```python
from build123d import *

# Parameters (mm, degrees)
BOX002_W     = 24
BOX002_H     = 2.4
BOX002_DEPTH = 20
BOX003_W     = 24
BOX003_H     = 2.4
BOX003_DEPTH = 20
BOX004_W     = 24
BOX004_H     = 2.4
BOX004_DEPTH = 20
BOX001_W     = 24
BOX001_H     = 2.4
BOX001_DEPTH = 20
BOX_W        = 30
BOX_H        = 33
BOX_DEPTH    = 22


with BuildPart() as box002:
    # Box002 → Box002 (new body)
    with BuildSketch(Plane(origin=(0, 5.6, 0), x_dir=(1, 0, 0), z_dir=(0, 0, 1))):
        with Locations((12, 1.2)):
            Rectangle(BOX002_W, BOX002_H)
    extrude(amount=BOX002_DEPTH)


with BuildPart() as box003:
    # Box003 → Box003 (new body)
    with BuildSketch(Plane(origin=(0, 11.2, 0), x_dir=(1, 0, 0), z_dir=(0, 0, 1))):
        with Locations((12, 1.2)):
            Rectangle(BOX003_W, BOX003_H)
    extrude(amount=BOX003_DEPTH)


with BuildPart() as box004:
    # Box004 → Box004 (new body)
    with BuildSketch(Plane(origin=(0, 16.8, 0), x_dir=(1, 0, 0), z_dir=(0, 0, 1))):
        with Locations((12, 1.2)):
            Rectangle(BOX004_W, BOX004_H)
    extrude(amount=BOX004_DEPTH)


with BuildPart() as ranuras:
    # Box001 → Box001 (new body)
    with BuildSketch(Plane.XY):
        with Locations((12, 1.2)):
            Rectangle(BOX001_W, BOX001_H)
    extrude(amount=BOX001_DEPTH)

    # Fusion: union Box002, Box003, Box004
    add(box002.part)
    add(box003.part)
    add(box004.part)


with BuildPart() as ranuras_1:
    # Fusion placement: moved
    add(ranuras.part.moved(Location((3, 7, 2))))


with BuildPart() as porta_sd:
    # Box → Box (new body)
    with BuildSketch(Plane.XY):
        with Locations((15, 16.5)):
            Rectangle(BOX_W, BOX_H)
    extrude(amount=BOX_DEPTH)

    # Cut: cut Ranuras
    add(ranuras_1.part, mode=Mode.SUBTRACT)


solid = porta_sd.part
```
Geometry: final body of the model. Coordinates: model frame, mm. A direction names the side the tool comes from. Give positions to 0.01 mm unless a question says otherwise; leave off trailing zeros. Order: outer loops, then holes, each group sorted by start corner. A loop starts at its lowest first (then second) coordinate and runs counter-clockwise, first axis right, second up. Notation, with made-up numbers: (56, -4) -> (89, -4) arc R6 cw to (89, 6) -> close; hole circle Ø11 at (78, 76). An arc over 180 degrees is marked (long way). Write each question's results on one line, items separated by ' | '. Start each with the question number.
1) Draft query along X for faces 3 (the flat face through (15, 0, 11)), 4 (the flat face through (0, 16, 11)), 5 (the flat face through (27, 19, 12)). Return one class per face: pulls with the +X half, pulls with the -X half, needs draft (parallel to the pull), parting line crosses it, or undercut.
2) First-contact query: pin 1 (1.9 mm diameter, centred on x = 17, y = 25, fed in from +Z). Flat tip, straight axial feed; report the tip coordinate or a pass-through.
3) Section C-C (x = 24.5). Return loops of the section in (y, z), then the cut area to 3 significant figures.
4) Set-up query: faces 1 (the flat face through (15, 23.8, 12)), 2 (the flat face through (15, 17, 22)). Return all of +Z, -Z, +X, -X, +Y, -Y with unobstructed straight access to the full face (end or side cutting, diameter ignored); none if empty.
5) Section A-A (z = 9.5). Return loops of the section in (x, y), then the cut area to 3 significant figures.
6) Line query: line 1 (Y direction, x = 11.5, z = 19); line 2 (X direction, y = 20.5, z = 13.25); line 3 (Z direction, x = 8.5, y = 7.5). Output: solid intervals per line, ascending. Write a range as from..to.
7) Section B-B (y = 14.5). Return loops of the section in (x, z).
Calculated:
1) face 3: needs draft | face 4: pulls with the -X half | face 5: undercut
2) pin 1: z = 2
3) outline: (0, 0) -> (33, 0) -> (33, 22) -> (26.2, 22) -> (26.2, 2) -> (23.8, 2) -> (23.8, 22) -> (20.6, 22) -> (20.6, 2) -> (18.2, 2) -> (18.2, 22) -> (15, 22) -> (15, 2) -> (12.6, 2) -> (12.6, 22) -> (9.4, 22) -> (9.4, 2) -> (7, 2) -> (7, 22) -> (0, 22) -> close | area: 534 mm2
4) face 1: +Z | face 2: +Z, +X, -X, +Y, -Y
5) outline: (0, 0) -> (30, 0) -> (30, 33) -> (0, 33) -> close; hole (3, 7) -> (27, 7) -> (27, 9.4) -> (3, 9.4) -> close; hole (3, 12.6) -> (27, 12.6) -> (27, 15) -> (3, 15) -> close; hole (3, 18.2) -> (27, 18.2) -> (27, 20.6) -> (3, 20.6) -> close; hole (3, 23.8) -> (27, 23.8) -> (27, 26.2) -> (3, 26.2) -> close | area: 760 mm2
6) line 1: 0..7, 9.4..12.6, 15..18.2, 20.6..23.8, 26.2..33 | line 2: 0..3, 27..30 | line 3: 0..2
7) outline: (0, 0) -> (30, 0) -> (30, 22) -> (27, 22) -> (27, 2) -> (3, 2) -> (3, 22) -> (0, 22) -> close
